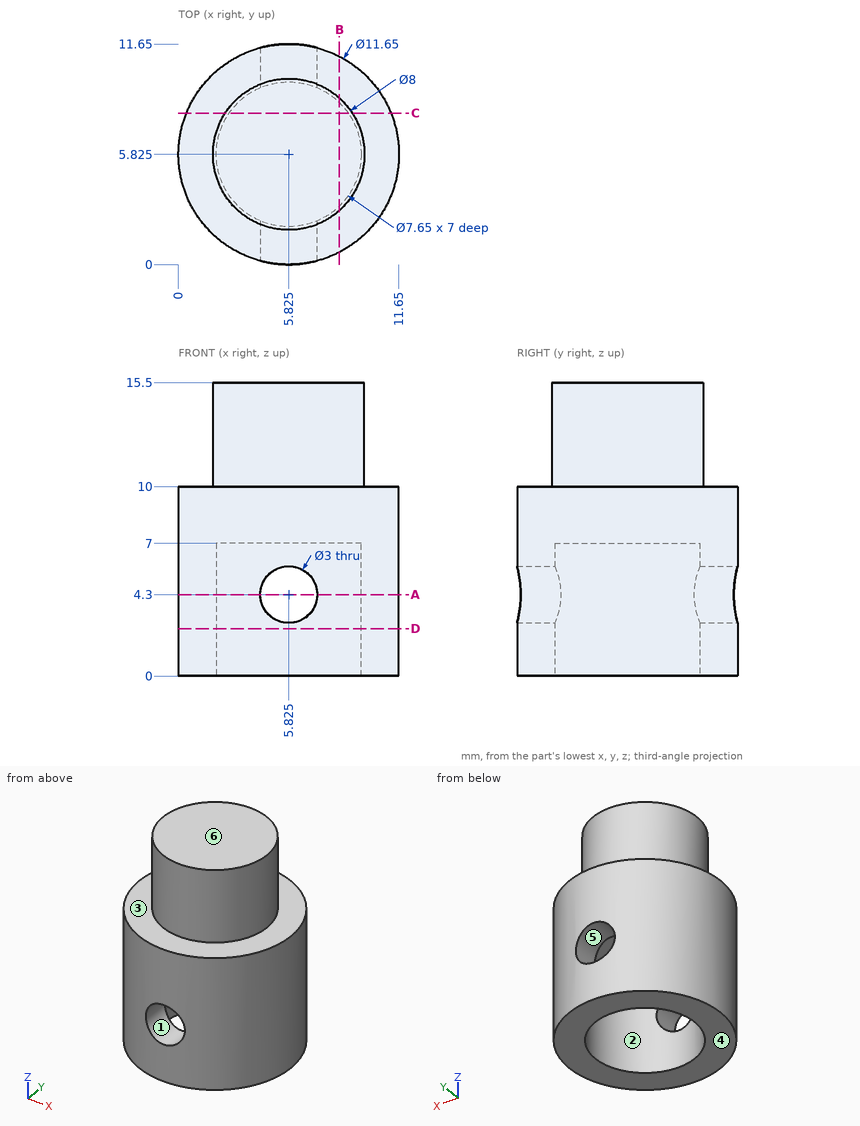
Geometry check sheet. Reference: drawing and pictorial views, mm from the part's lowest x, y, z. A direction names the side the tool comes from. Round coordinates to 2 decimals unless told otherwise and drop trailing zeros. Loops run counter-clockwise (first coordinate to the right, second up) from the corner with the lowest first, then second, coordinate; pieces in that order, holes last. Notation, with made-up numbers: (70, 18.5) - (106, 18.5) arc R19 ccw to (106, 47.5) - close; hole circle Ø9 at (89, 19.5). An arc over 180 degrees is marked (long way). Answer in a Markdown table with one row per item. Add a question column.
Q1. Section check B-B on x = 8.5. Enter the section's corners in (y, z), plus the area to 3 significant figures.
Q2. Material ranges on line 1 (Z direction, x = 5, y = 6.5); line 2 (Z direction, x = 8.75, y = 9.75); line 3 (Y direction, x = 3.5, z = 5.5), recorded low to high.
Q3. Release check for a two-part mould opening along Z. For the marked faces 4, 5 and 6 record: pulls with the +Z half, pulls with the -Z half, needs draft (parallel to the pull), parting line crosses it, or undercut.
Q4. Section check C-C on y = 8. Enter the section's corners in (x, z).
Q5. Tool access check on the marked faces 1, 2 and 3. Record the directions out of +Z, -Z, +X, -X, +Y, -Y that give a thin tool (end or side, any length) a straight path to the whole face; none if there is none.
Q6. Gauge pin test, flat ends, axial feed: pin 1 (6 mm diameter, centred on y = 9, z = 2.5, fed in from -X); pin 2 (6 mm diameter, centred on x = 6.5, z = 11.5, fed in from +Y); pin 3 (1.5 mm diameter, centred on y = 4, z = 12.5, fed in from -X); pin 4 (1 mm diameter, centred on x = 7, y = 4.5, fed in from -Z). Record the tip position at first contact, or that the pin passes through.
Q7. Section check A-A on z = 4.3. Enter the section's corners in (x, y) (3 decimals), plus the area to 3 significant figures.
Q8. Section check D-D on z = 2.5. Enter the section's corners in (x, y) (3 decimals), plus the area to 3 significant figures.
Found:
| question | item | result |
|---|---|---|
| 1 | outline | (0.65, 0) - (3.09, 0) - (3.09, 7) - (8.56, 7) - (8.56, 0) - (11, 0) - (11, 10) - (8.8, 10) - (8.8, 15.5) - (2.85, 15.5) - (2.85, 10) - (0.65, 10) - close |
| 1 | area | 97.9 mm² |
| 2 | line 1 | z = 7 to 15.5 |
| 2 | line 2 | z = 0 to 10 |
| 2 | line 3 | y = 0.48 to 2.79, 8.86 to 11.17 |
| 3 | face 4 | pulls with the -Z half |
| 3 | face 5 | undercut |
| 3 | face 6 | pulls with the +Z half |
| 4 | outline | (0.42, 0) - (2.68, 0) - (2.68, 7) - (8.97, 7) - (8.97, 0) - (11.23, 0) - (11.23, 10) - (9.18, 10) - (9.18, 15.5) - (2.47, 15.5) - (2.47, 10) - (0.42, 10) - close |
| 5 | face 1 | +Y, -Y |
| 5 | face 2 | -Z |
| 5 | face 3 | +Z |
| 6 | pin 1 | stops at x = 0 |
| 6 | pin 2 | stops at y = 11.65 |
| 6 | pin 3 | stops at x = 1.97 |
| 6 | pin 4 | stops at z = 7 |
| 7 | outline | (4.325, 0.196) - (4.325, 2.306) arc R3.825 cw to (4.325, 9.344) - (4.325, 11.454) arc R5.825 ccw to start; (7.325, 0.196) arc R5.825 ccw to (7.325, 11.454) - (7.325, 9.344) arc R3.825 cw to (7.325, 2.306) - close |
| 7 | area | 48.4 mm² |
| 8 | outline | circle Ø11.65 at (5.825, 5.825); hole circle Ø7.65 at (5.825, 5.825) |
| 8 | area | 60.6 mm² |
